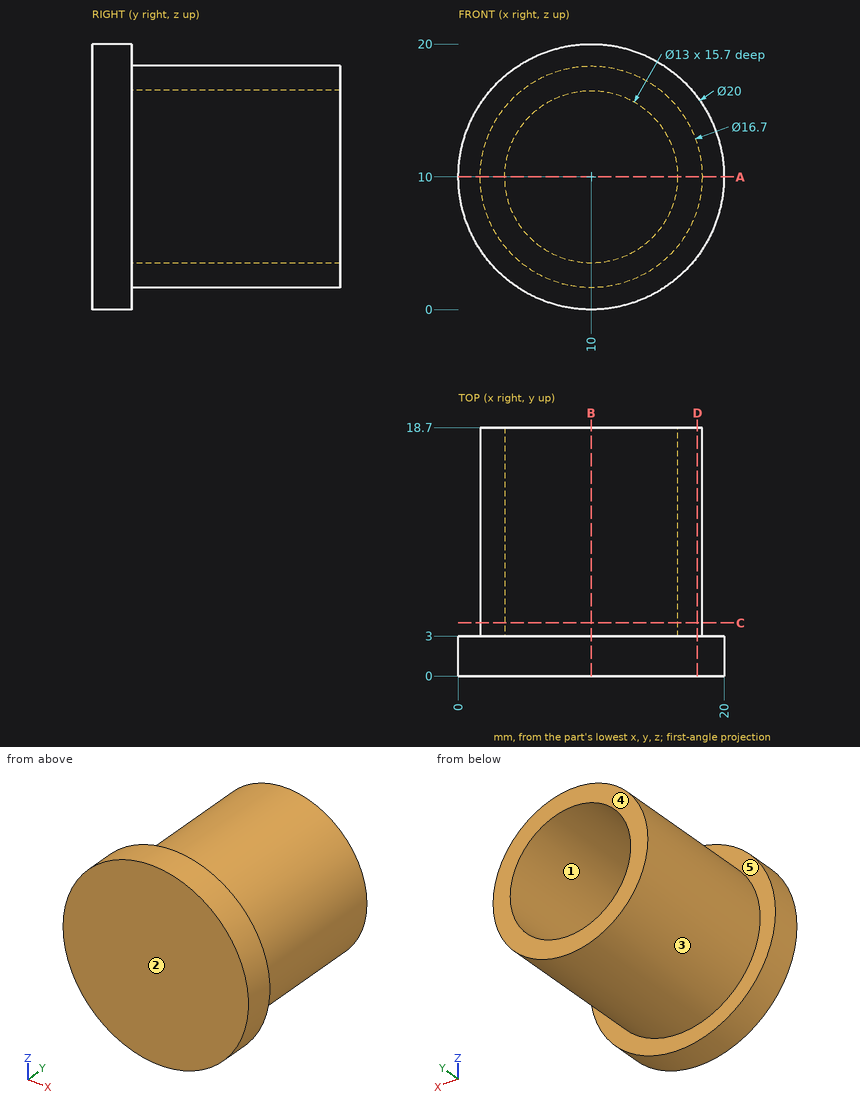
The figure shows three views and two pictorial views of one solid part (mm, origin at its lowest corner). Answer the questions. A direction names the side the tool comes from. Give positions to 0.01 mm unless a question says otherwise; leave off trailing zeros. Write each loop counter-clockwise with the first axis right and the second up, starting at its lowest first coordinate (ties: lowest second). Pieces come first, ordered by that corner, then holes. Notation, with made-up numbers: M -7.5,26.5 L 43.5,26.5 A20 cw 43.5,45.5 Z; hole C -16.75,41.25 d10. An arc over 180 degrees is marked long. Write each question's results on one line, items separated by ' | '.
Q1. A tool of negligible diameter and unlimited length cuts with its end or side. For the marked faces 4 and 5, from which of +Z, -Z, +X, -X, +Y, -Y can it reach the whole face along a straight path? Write none if from no direction.
Output values:
face 4: +Z, -Z, +X, -X, +Y | face 5: +Y
Q2. For a pull along Z with two mould halves and no side action, classify the marked faces 1, 2 and 3 as released by +Z, released by -Z, zero draft, split by the parting line, or undercut.
Output values:
face 1: undercut | face 2: zero draft | face 3: split by the parting line
Q3. Flat-ended cylindrical pins translate along their axes: P1, Ø2, axis at x = 13, y = 7, coming from the -Z side; P2, Ø10, axis at y = 14.5, z = 8.5, coming from the +X side; P3, Ø1, axis at x = 12.5, y = 13, coming from the +Z side. Find the tip coordinate at first contact, or state that the pin passes through.
Output values:
P1: z = 1.89 | P2: x = 18.35 | P3: z = 18.11
Q4. Section C-C, the plane y = 4 is taken. Write down the section's boundary in (x, z).
Output values:
outline: C 10,10 d16.7; hole C 10,10 d13
Q5. Section D-D, the plane x = 18 is taken. Write down the section's boundary in (y, z), then the cut area to 3 significant figures.
Output values:
outline: M 0,4 L 3,4 L 3,7.61 L 18.7,7.61 L 18.7,12.39 L 3,12.39 L 3,16 L 0,16 Z | area: 111 mm2
Q6. Consider L1, parallel to X at y = 14.5, z = 10; L2, parallel to Y at x = 5, z = 12. Determine where each line is inside the solid, lowest interval first. Write a range as from..to.
Output values:
L1: 1.65..3.5, 16.5..18.35 | L2: 0..3
Q7. Section B-B, the plane x = 10 is taken. Write down the section's boundary in (y, z).
Output values:
outline: M 0,0 L 3,0 L 3,1.65 L 18.7,1.65 L 18.7,3.5 L 3,3.5 L 3,16.5 L 18.7,16.5 L 18.7,18.35 L 3,18.35 L 3,20 L 0,20 Z
Q8. Section A-A, the plane z = 10 is taken. Write down the section's boundary in (x, y).
Output values:
outline: M 0,0 L 20,0 L 20,3 L 18.35,3 L 18.35,18.7 L 16.5,18.7 L 16.5,3 L 3.5,3 L 3.5,18.7 L 1.65,18.7 L 1.65,3 L 0,3 Z
